Geometry: see drawing. Coordinates: mm, zero at the bounding-box minimum. Coordinates: 2 decimals unless noted, no trailing zeros. One line per question, with ' | ' between items. Start each with the question number.
1. Pin query (flat end, axial travel): P1, Ø11, axis at x = 66.971, y = 44.45, coming from the +Z side; P2, Ø13.5, axis at x = 21.971, y = 44.45, coming from the +Z side; P3, Ø4, axis at x = 42.5, y = 13, coming from the -Z side. Return the tip coordinate at first contact, or that it passes through.
2. Mould query, pull axis Y, two halves, no side actions, for the marked faces 1 and 2. Classes: pulls with the +Y half, pulls with the -Y half, needs draft (parallel to the pull), parting line crosses it, or undercut.
3. Section query A-A, the plane y = 44.45. State how many separate pieces and enclosed holes the cut face has, and give its area (3 significant figures).
4. Ray query, probe 1 along X at (y, z) = (44.45, 1) (1 decimal); probe 2 along X at (y, z) = (47, 4) (1 decimal); probe 3 along Y at (x, z) = (18, 6.25). Return the intervals inside material, ascending.
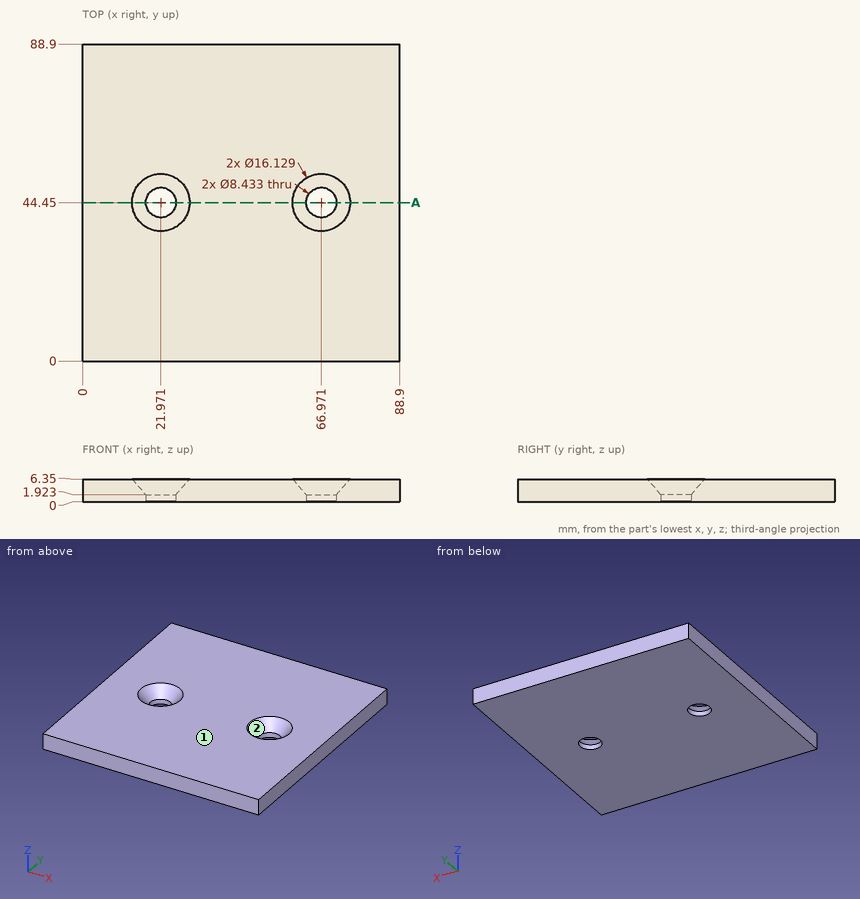
Taken from the geometry:
1) P1: z = 3.4 | P2: z = 4.84 | P3: z = 0
2) face 1: needs draft | face 2: undercut
3) separate pieces: 3 | enclosed holes: 0 | area: 423 mm^2
4) probe 1: 0 to 17.8, 26.2 to 62.8, 71.2 to 88.9 | probe 2: 0 to 16.5, 27.4 to 61.5, 72.4 to 88.9 | probe 3: 0 to 37.53, 51.37 to 88.9
